Part model, mm, in its own coordinate system. Round coordinates to 2 decimals unless told otherwise and drop trailing zeros. Loops run counter-clockwise (first coordinate to the right, second up) from the corner with the lowest first, then second, coordinate; pieces in that order, holes last.
from build123d import *

# Parameters (mm, degrees)
SKETCH1_W               = 152.4
SKETCH1_H               = 127
BOSS_EXTRUDE1_DEPTH     = 3.175
FILLET1_R               = 2.54
SKETCH9_R               = 4.15
CUT_EXTRUDE8_DEPTH      = 100.240972511
CUT_EXTRUDE11_DEPTH     = 100.240972511
CUT_EXTRUDE12_DEPTH     = 100.240972511
SKETCH15_R              = 4.15
CUT_EXTRUDE13_DEPTH     = 100.240972511
SKETCH16_R              = 4.15
CUT_EXTRUDE14_DEPTH     = 100.240972511
SKETCH17_R              = 2.69
CUT_EXTRUDE16_DEPTH     = 100.240972511
MIRROR7_COPY_1_SKETCH_R = 2.69
MIRROR7_COPY_1_DEPTH    = 100.240972511
SKETCH18_R              = 4.15
CUT_EXTRUDE17_DEPTH     = 100.240972511
SKETCH19_R              = 4.15
CUT_EXTRUDE18_DEPTH     = 100.240972511
SKETCH20_R              = 4.15
CUT_EXTRUDE19_DEPTH     = 100.240972511
SKETCH21_W              = 7.62
SKETCH21_H              = 13.958580006
CUT_EXTRUDE20_DEPTH     = 100.240972511
SKETCH22_W              = 15.228595593
SKETCH22_H              = 53.32954849
SKETCH22_W_2            = 12.7
SKETCH22_H_2            = 50.8
CUT_EXTRUDE21_DEPTH     = 0.79375
SKETCH24_W              = 21.59
SKETCH24_H              = 53.34
SKETCH24_W_2            = 19.05
SKETCH24_H_2            = 50.8
CUT_EXTRUDE24_DEPTH     = 0.79375


with BuildPart() as part:
    # Sketch1 → Boss-Extrude1 (new body)
    with BuildSketch(Plane(origin=(0, 0, 0), x_dir=(1, 0, 0), z_dir=(0, 1, 0))):
        Rectangle(SKETCH1_W, SKETCH1_H)
    extrude(amount=BOSS_EXTRUDE1_DEPTH)

    # Fillet1
    fillet1_edges = [part.edges().sort_by_distance(p)[0] for p in [
        (76.2, 1.5875, 63.5),
        (-76.2, 1.5875, 63.5),
        (-76.2, 1.5875, -63.5),
        (76.2, 1.5875, -63.5),
    ]]
    fillet(fillet1_edges, radius=FILLET1_R)

    # Sketch9 → Cut-Extrude8 (cut, through all)
    with BuildSketch(Plane.XZ):
        with Locations(Location((60.8584, 30.027977178, 0), (0, 0, 270))):
            Circle(SKETCH9_R)
        with Locations(Location((60.8584, -0.452022822, 0), (0, 0, 270))):
            Circle(SKETCH9_R)
    extrude(amount=-CUT_EXTRUDE8_DEPTH, mode=Mode.SUBTRACT)

    # Sketch12 → Cut-Extrude11 (cut, through all)
    with BuildSketch(Plane.XZ):
        with BuildLine():
            Line((-3.81, 59.465627528), (3.81, 59.465627528))
            ThreePointArc((3.81, 59.465627528), (8.387405636, 54.888221892), (3.81, 50.310816255))
            Line((3.81, 50.310816255), (-3.81, 50.310816255))
            ThreePointArc((-3.81, 50.310816255), (-8.387405636, 54.888221892), (-3.81, 59.465627528))
        make_face()
    cut_extrude11 = extrude(amount=-CUT_EXTRUDE11_DEPTH, mode=Mode.SUBTRACT)

    # Mirror3: Cut-Extrude11 across plane
    add(cut_extrude11.mirror(Plane.XY), mode=Mode.SUBTRACT)

    # Sketch13 → Cut-Extrude12 (cut, through all)
    with BuildSketch(Plane(origin=(0, 0, 0), x_dir=(-1, 0, 0), z_dir=(0, -1, 0))):
        with BuildLine():
            Line((49.892874771, -36.83), (49.892874771, -44.45))
            ThreePointArc((49.892874771, -44.45), (45.72, -48.622874771), (41.547125229, -44.45))
            Line((41.547125229, -44.45), (41.547125229, -36.83))
            ThreePointArc((41.547125229, -36.83), (45.72, -32.657125229), (49.892874771, -36.83))
        make_face()
    extrude(amount=-CUT_EXTRUDE12_DEPTH, mode=Mode.SUBTRACT)

    # Sketch15 → Cut-Extrude13 (cut, through all)
    with BuildSketch(Plane(origin=(0, 0, 0), x_dir=(-1, 0, 0), z_dir=(0, -1, 0))):
        with Locations(Location((41.916131811, 18.596838804, 0), (0, 0, 90))):
            Circle(SKETCH15_R)
        with Locations(Location((41.916131811, -18.596838804, 0), (0, 0, 90))):
            Circle(SKETCH15_R)
    extrude(amount=-CUT_EXTRUDE13_DEPTH, mode=Mode.SUBTRACT)

    # Sketch16 → Cut-Extrude14 (cut, through all)
    with BuildSketch(Plane(origin=(0, 0, 0), x_dir=(-1, 0, 0), z_dir=(0, -1, 0))):
        with Locations(Location((-69.599893995, 30.499477113, 0), (0, 0, 90))):
            Circle(SKETCH16_R)
        with Locations(Location((-46.522565834, 43.05939533, 0), (0, 0, 90))):
            Circle(SKETCH16_R)
    extrude(amount=-CUT_EXTRUDE14_DEPTH, mode=Mode.SUBTRACT)

    # Sketch17 → Cut-Extrude16 (cut, through all)
    with BuildSketch(Plane.XZ):
        with Locations(Location((72.867806522, 60.482193478, 0), (0, 0, 270))):
            Circle(SKETCH17_R)
    cut_extrude16 = extrude(amount=-CUT_EXTRUDE16_DEPTH, mode=Mode.SUBTRACT)

    # Mirror6: Cut-Extrude16 across plane
    add(cut_extrude16.mirror(Plane(origin=(0, 0, 0), x_dir=(0, 0, 1), z_dir=(1, 0, 0))), mode=Mode.SUBTRACT)

    # Mirror7: Cut-Extrude16 across plane
    add(cut_extrude16.mirror(Plane.XY), mode=Mode.SUBTRACT)

    # Mirror7 copy 1 sketch → Mirror7 copy 1 (cut, through all)
    with BuildSketch(Plane(origin=(0, 0, 0), x_dir=(-1, 0, 0), z_dir=(0, -1, 0))):
        with Locations(Location((72.867806522, 60.482193478, 0), (0, 0, 270))):
            Circle(MIRROR7_COPY_1_SKETCH_R)
    extrude(amount=-MIRROR7_COPY_1_DEPTH, mode=Mode.SUBTRACT)

    # Sketch18 → Cut-Extrude17 (cut, through all)
    with BuildSketch(Plane(origin=(0, 3.175, 0), x_dir=(1, 0, 0), z_dir=(0, 1, 0))):
        with Locations(Location((37.078939717, 21.853932791, 0), (0, 0, 270))):
            Circle(SKETCH18_R)
        with Locations(Location((37.078939717, -17.508548393, 0), (0, 0, 270))):
            Circle(SKETCH18_R)
    extrude(amount=-CUT_EXTRUDE17_DEPTH, mode=Mode.SUBTRACT)

    # Sketch19 → Cut-Extrude18 (cut, through all)
    with BuildSketch(Plane(origin=(0, 3.175, 0), x_dir=(1, 0, 0), z_dir=(0, 1, 0))):
        with Locations(Location((52.190187574, -56.270763327, 0), (0, 0, 270))):
            Circle(SKETCH19_R)
        with Locations(Location((18.821046034, -56.270763327, 0), (0, 0, 270))):
            Circle(SKETCH19_R)
    cut_extrude18 = extrude(amount=-CUT_EXTRUDE18_DEPTH, mode=Mode.SUBTRACT)

    # Sketch20 → Cut-Extrude19 (cut, through all)
    with BuildSketch(Plane(origin=(0, 3.175, 0), x_dir=(1, 0, 0), z_dir=(0, 1, 0))):
        with Locations(Location((-62.798787331, 12.836349908, 0), (0, 0, 270))):
            Circle(SKETCH20_R)
        with Locations(Location((-62.798787331, -13.535650092, 0), (0, 0, 270))):
            Circle(SKETCH20_R)
    extrude(amount=-CUT_EXTRUDE19_DEPTH, mode=Mode.SUBTRACT)

    # Mirror8: Cut-Extrude18 across plane
    add(cut_extrude18.mirror(Plane.XY), mode=Mode.SUBTRACT)

    # Sketch21 → Cut-Extrude20 (cut, through all)
    with BuildSketch(Plane.XZ):
        with Locations((37.078939717, -2.172692199)):
            Rectangle(SKETCH21_W, SKETCH21_H)
    extrude(amount=-CUT_EXTRUDE20_DEPTH, mode=Mode.SUBTRACT)

    # Sketch22 → Cut-Extrude21 (cut)
    with BuildSketch(Plane(origin=(0, 3.175, 0), x_dir=(1, 0, 0), z_dir=(0, 1, 0))):
        with Locations((-41.904297797, 0.005225755)):
            Rectangle(SKETCH22_W, SKETCH22_H)
        with Locations((-41.91, 0)):
            Rectangle(SKETCH22_W_2, SKETCH22_H_2, mode=Mode.SUBTRACT)
    extrude(amount=-CUT_EXTRUDE21_DEPTH, mode=Mode.SUBTRACT)

    # Sketch24 → Cut-Extrude24 (cut)
    with BuildSketch(Plane(origin=(0, 3.175, 0), x_dir=(-1, 0, 0), z_dir=(0, -1, 0))):
        with Locations((-60.8584, -14.787977178)):
            Rectangle(SKETCH24_W, SKETCH24_H)
        with Locations((-60.8584, -14.787977178)):
            Rectangle(SKETCH24_W_2, SKETCH24_H_2, mode=Mode.SUBTRACT)
    extrude(amount=CUT_EXTRUDE24_DEPTH, mode=Mode.SUBTRACT)


solid = part.part
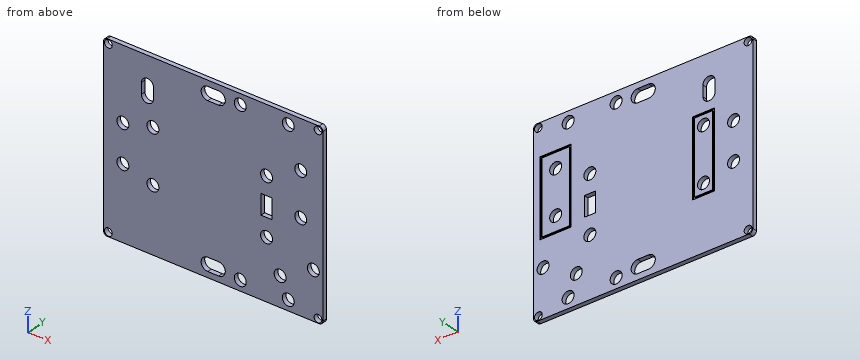
1) Wall check: line 1 along X through (y, z) = (0.35, -0.5); line 2 along Z through (x, y) = (-2.5, 2.3); line 3 along Z through (x, y) = (-43, 2.1). Give the ranges that are in metal, low to high.
Values:
line 1: x = -76.2 to 33.27, 40.89 to 56.71, 65.01 to 76.2
line 2: z = -63.5 to -59.47, -50.31 to 50.31, 59.47 to 63.5
line 3: z = -63.5 to -22.6, -14.59 to 14.59, 22.6 to 33.67, 47.61 to 63.5
2) Drop flat-ended pins along their axis: pin 1 Ø7.5 at (x, z) = (46.52, -43.06) entering from +Y; pin 2 Ø10 at (x, z) = (3, -12) entering from -Y. Give the stop position or say it passes through.
Values:
pin 1: passes through
pin 2: stops at y = 0
3) Slice it at B-B, the plane y = 1.05. Give the number of separate pieces and of enclosed holes in the cut face, then the cut area to 3 significant figures.
Values:
separate pieces: 1
enclosed holes: 22
area: 18,000 mm2
4) Slice it at A-A, the plane x = -60.5. Give the cut face in (y, z) (1 decimal).
Values:
outline: (0, -63.5) - (3.2, -63.5) - (3.2, -16.3) - (0, -16.3) - close; (0, -9.4) - (3.2, -9.4) - (3.2, 10.1) - (0, 10.1) - close; (0, 17) - (3.2, 17) - (3.2, 63.5) - (0, 63.5) - close
